from build123d import *

# Parameters (mm, degrees)
SKIZZE1_R                            = 25.1
SKIZZE1_W                            = 20
SKIZZE1_H                            = 20
AUFSATZ_LINEAR_AUSTRAGEN1_DEPTH      = 15
SKIZZE2_R                            = 25.1
SKIZZE2_R_2                          = 23.6
AUFSATZ_LINEAR_AUSTRAGEN2_DEPTH      = 3.6
SKIZZE3_R                            = 2
SCHNITT_LINEAR_AUSTRAGEN2_DEPTH      = 19.6
SKIZZE4_R                            = 2.7
SCHNITT_LINEAR_AUSTRAGEN3_DEPTH      = 26.1
SCHNITT_LINEAR_AUSTRAGEN3_DEPTH_BACK = 26.1
SKIZZE5_R                            = 2.7
SCHNITT_LINEAR_AUSTRAGEN4_DEPTH      = 26.1000001
SCHNITT_LINEAR_AUSTRAGEN4_DEPTH_BACK = 26.1000001
SCHNITT_LINEAR_START                 = 13
SKIZZE4_3_R                          = 5
SCHNITT_LINEAR_AUSTRAGEN5_DEPTH      = 13.1000001
SKIZZE5_3_R                          = 5
SCHNITT_LINEAR_AUSTRAGEN6_DEPTH      = 13.1000001


with BuildPart() as part:
    # Skizze1 → Aufsatz-Linear austragen1 (new body)
    with BuildSketch(Plane.XY):
        Circle(SKIZZE1_R)
        Rectangle(SKIZZE1_W, SKIZZE1_H, mode=Mode.SUBTRACT)
    extrude(amount=AUFSATZ_LINEAR_AUSTRAGEN1_DEPTH)

    # Skizze2 → Aufsatz-Linear austragen2 (add)
    with BuildSketch(Plane.XY.offset(15)):
        Circle(SKIZZE2_R)
        Circle(SKIZZE2_R_2, mode=Mode.SUBTRACT)
    extrude(amount=AUFSATZ_LINEAR_AUSTRAGEN2_DEPTH)

    # Skizze3 → Schnitt-Linear austragen2 (cut, through all)
    with BuildSketch(Plane.XY):
        with Locations((-10, 10)):
            Circle(SKIZZE3_R)
        with Locations((10, 10)):
            Circle(SKIZZE3_R)
        with Locations((10, -10)):
            Circle(SKIZZE3_R)
        with Locations((-10, -10)):
            Circle(SKIZZE3_R)
    extrude(amount=SCHNITT_LINEAR_AUSTRAGEN2_DEPTH, mode=Mode.SUBTRACT)

    # Skizze4 → Schnitt-Linear austragen3 (cut, two sides)
    with BuildSketch(Plane(origin=(0, 0, 0), x_dir=(1, 0, 0), z_dir=(0, 1, 0))) as schnitt_linear_austragen3_sk:
        with Locations((0, -7.5)):
            Circle(SKIZZE4_R)
    extrude(amount=SCHNITT_LINEAR_AUSTRAGEN3_DEPTH, mode=Mode.SUBTRACT)
    extrude(schnitt_linear_austragen3_sk.sketch, amount=-SCHNITT_LINEAR_AUSTRAGEN3_DEPTH_BACK, mode=Mode.SUBTRACT)

    # Skizze5 → Schnitt-Linear austragen4 (cut, two sides)
    with BuildSketch(Plane(origin=(0, 0, 0), x_dir=(0, 0, -1), z_dir=(1, 0, 0))) as schnitt_linear_austragen4_sk:
        with Locations((-7.5, 0)):
            Circle(SKIZZE5_R)
    extrude(amount=SCHNITT_LINEAR_AUSTRAGEN4_DEPTH, mode=Mode.SUBTRACT)
    extrude(schnitt_linear_austragen4_sk.sketch, amount=-SCHNITT_LINEAR_AUSTRAGEN4_DEPTH_BACK, mode=Mode.SUBTRACT)

    # Skizze4<3> → Schnitt-Linear austragen5 (cut, through all)
    with BuildSketch(Plane(origin=(0, 0, 0), x_dir=(1, 0, 0), z_dir=(0, 1, 0)).offset(SCHNITT_LINEAR_START)):
        with Locations((0, -7.5)):
            Circle(SKIZZE4_3_R)
    schnitt_linear_austragen5 = extrude(amount=SCHNITT_LINEAR_AUSTRAGEN5_DEPTH, mode=Mode.SUBTRACT)

    # Spiegeln1: Schnitt-Linear austragen5 across plane
    add(schnitt_linear_austragen5.mirror(Plane.ZX), mode=Mode.SUBTRACT)

    # Skizze5<3> → Schnitt-Linear austragen6 (cut, through all)
    with BuildSketch(Plane(origin=(0, 0, 0), x_dir=(0, 0, -1), z_dir=(1, 0, 0)).offset(SCHNITT_LINEAR_START)):
        with Locations((-7.5, 0)):
            Circle(SKIZZE5_3_R)
    schnitt_linear_austragen6 = extrude(amount=SCHNITT_LINEAR_AUSTRAGEN6_DEPTH, mode=Mode.SUBTRACT)

    # Spiegeln2: Schnitt-Linear austragen6 across plane
    add(schnitt_linear_austragen6.mirror(Plane(origin=(0, 0, 0), x_dir=(0, 0, 1), z_dir=(1, 0, 0))), mode=Mode.SUBTRACT)


solid = part.part
The model under review builds one solid part; all positions refer to its coordinate system, in mm. A direction names the side the tool comes from. Give positions to 0.01 mm unless a question says otherwise; leave off trailing zeros. Write each loop counter-clockwise with the first axis right and the second up, starting at its lowest first coordinate (ties: lowest second). Pieces come first, ordered by that corner, then holes.
1. Add section D-D, the plane y = -7. Write out the cut boundary in (x, z).
2. Tool access review of faces 1 (the cylindrical face through (-23.577, 1.038, 16.775)), 2 (the cylindrical face through (-0.651, 18.965, 2.543)), 3 (the flat face through (13, -2, 5)): name each direction out of +Z, -Z, +X, -X, +Y, -Y from which nothing blocks a thin tool from reaching the whole face with its end or side.
3. Draft analysis for pull direction Y (two halves, no side actions). For faces 4 (the cylindrical face through (23.186, -9.613, 9.17)), 5 (the cylindrical face through (-11.479, -1.643, 9.643)), 6 (the cylindrical face through (-0.585, -11.479, 10.136)), state which applies: +Y half, -Y half, draft (parallel to the pull), parting line (faces both ways), or undercut.
4. Wall thickness on L1, parallel to Z at x = 0, y = -11; L2, parallel to X at y = 1, z = 12; L3, parallel to Y at x = 11, z = 13.75: over which ranges is each line inside the solid? List them lowest first.
5. Add section A-A, the plane y = 0. Write out the cut boundary in (x, z).
6. Add section C-C, the plane x = -18. Write out the cut boundary in (y, z).
7. For P1, Ø8, axis at x = 2.5, z = 7, coming from the -Y side; P2, Ø1, axis at x = 17.5, z = 14.5, coming from the -Y side; P3, Ø6, axis at x = 0, z = 7.5, coming from the +Y side; P4, Ø3, axis at x = 0, z = 7.5, coming from the +Y side, all flat-tipped, find the tip position at first contact; note any pin that passes through.
Worked answers:
1. outline: (-24.1, 0) - (-10, 0) - (-10, 15) - (-22.54, 15) - (-22.54, 18.6) - (-24.1, 18.6) - close; (10, 0) - (24.1, 0) - (24.1, 18.6) - (22.54, 18.6) - (22.54, 15) - (10, 15) - close
2. face 1: +Z
2. face 2: +Y
2. face 3: +X
3. face 4: parting line
3. face 5: undercut
3. face 6: draft
4. L1: z = 0 to 4.8, 10.2 to 15
4. L2: x = -13 to -10, 10 to 13
4. L3: y = -22.56 to -11.73, -8.27 to 8.27, 11.73 to 22.56
5. outline: (-25.1, 0) - (-10, 0) - (-10, 4.8) - (-13, 4.8) - (-13, 2.5) - (-25.1, 2.5) - close; (-25.1, 12.5) - (-13, 12.5) - (-13, 10.2) - (-10, 10.2) - (-10, 15) - (-23.6, 15) - (-23.6, 18.6) - (-25.1, 18.6) - close; (10, 0) - (25.1, 0) - (25.1, 2.5) - (13, 2.5) - (13, 4.8) - (10, 4.8) - close; (10, 10.2) - (13, 10.2) - (13, 12.5) - (25.1, 12.5) - (25.1, 18.6) - (23.6, 18.6) - (23.6, 15) - (10, 15) - close
6. outline: (-17.49, 0) - (17.49, 0) - (17.49, 18.6) - (15.26, 18.6) - (15.26, 15) - (-15.26, 15) - (-15.26, 18.6) - (-17.49, 18.6) - close; hole circle Ø10 at (0, 7.5)
7. P1: stops at y = -25
7. P2: stops at y = -18.47
7. P3: stops at y = 13
7. P4: passes through
